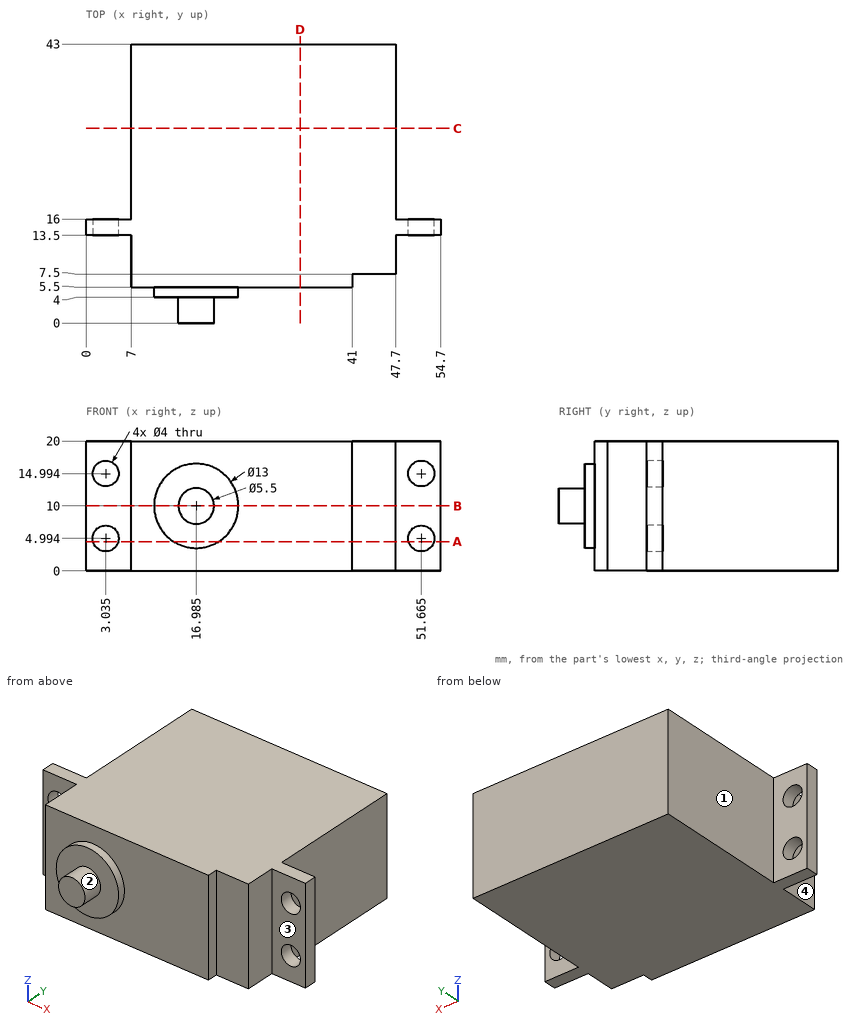
Design review of the part shown in the three views and the two pictorial views. Dimensions are in mm from the part's minimum x, y and z. A direction names the side the tool comes from. Give positions to 0.01 mm unless a question says otherwise; leave off trailing zeros. Order: outer loops, then holes, each group sorted by start corner. A loop starts at its lowest first (then second) coordinate and runs counter-clockwise, first axis right, second up. Notation, with made-up numbers: (53, 82.5) -> (90, 82.5) arc R13 ccw to (90, 86.5) -> close; hole circle Ø3 at (-32.75, 84.5). An arc over 180 degrees is marked (long way). Write each question's results on one line, items separated by ' | '. Start each with the question number.
Q1. Add section C-C on y = 30. Give the boundary of the cut face in (x, z), and give its area (3 significant figures).
Q2. Add section A-A on z = 4.5. Give the boundary of the cut face in (x, y).
Q3. Machinability: for the marked faces 1, 2, 3 and 4, which of the approach directions +Z, -Z, +X, -X, +Y, -Y give a long, thin tool a straight path to every point of the face, cutting with its end or side? Answer none if there is none.
Q4. Wall thickness on L1, parallel to Y at x = 47, z = 11.75; L2, parallel to Y at x = 24.5, z = 6.5; L3, parallel to X at y = 24, z = 14: over which ranges is each line inside the solid? List them lowest first. Write a range as from..to.
Q5. Add section B-B on z = 10. Give the boundary of the cut face in (x, y) (1 decimal).
Q6. Add section D-D on x = 33. Give the boundary of the cut face in (y, z), and give its area (3 significant figures).
Q7. For pin 1 (3.5 mm diameter, centred on x = 4.5, z = 5.5, fed in from -Y); pin 2 (1 mm diameter, centred on y = 30, z = 18, fed in from -X); pin 3 (4 mm diameter, centred on y = 9.5, z = 9.5, fed in from +X), all flat-tipped, find the tip position at first contact; note any pin that passes through.
Found:
1) outline: (7, 0) -> (47.7, 0) -> (47.7, 20) -> (7, 20) -> close | area: 814 mm2
2) outline: (0, 13.5) -> (1.1, 13.5) -> (1.1, 16) -> (0, 16) -> close; (4.97, 13.5) -> (7, 13.5) -> (7, 5.5) -> (13.52, 5.5) -> (13.52, 4) -> (20.45, 4) -> (20.45, 5.5) -> (41, 5.5) -> (41, 7.5) -> (47.7, 7.5) -> (47.7, 13.5) -> (49.73, 13.5) -> (49.73, 16) -> (47.7, 16) -> (47.7, 43) -> (7, 43) -> (7, 16) -> (4.97, 16) -> close; (53.6, 13.5) -> (54.7, 13.5) -> (54.7, 16) -> (53.6, 16) -> close
3) face 1: +Z, -Z, -X, +Y | face 2: -Y | face 3: +Z, -Z, +X, -Y | face 4: +Z, -Z, -X, -Y
4) L1: y = 7.5..43 | L2: y = 5.5..43 | L3: x = 7..47.7
5) outline: (0, 13.5) -> (7, 13.5) -> (7, 5.5) -> (10.5, 5.5) -> (10.5, 4) -> (14.2, 4) -> (14.2, 0) -> (19.7, 0) -> (19.7, 4) -> (23.5, 4) -> (23.5, 5.5) -> (41, 5.5) -> (41, 7.5) -> (47.7, 7.5) -> (47.7, 13.5) -> (54.7, 13.5) -> (54.7, 16) -> (47.7, 16) -> (47.7, 43) -> (7, 43) -> (7, 16) -> (0, 16) -> close
6) outline: (5.5, 0) -> (43, 0) -> (43, 20) -> (5.5, 20) -> close | area: 750 mm2
7) pin 1: stops at y = 13.5 | pin 2: stops at x = 7 | pin 3: stops at x = 47.7
